Geometry check sheet. Reference: drawing and pictorial views, mm from the part's lowest x, y, z. A direction names the side the tool comes from. Coordinates: 2 decimals unless noted, no trailing zeros. Loops run counter-clockwise (first coordinate to the right, second up) from the corner with the lowest first, then second, coordinate; pieces in that order, holes last. Notation, with made-up numbers: (12.25, 54) - (60.25, 54) arc R22 cw to (60.25, 71) - close; hole circle Ø2 at (-23.5, 66.25). An arc over 180 degrees is marked (long way). One line per item, written item: value.
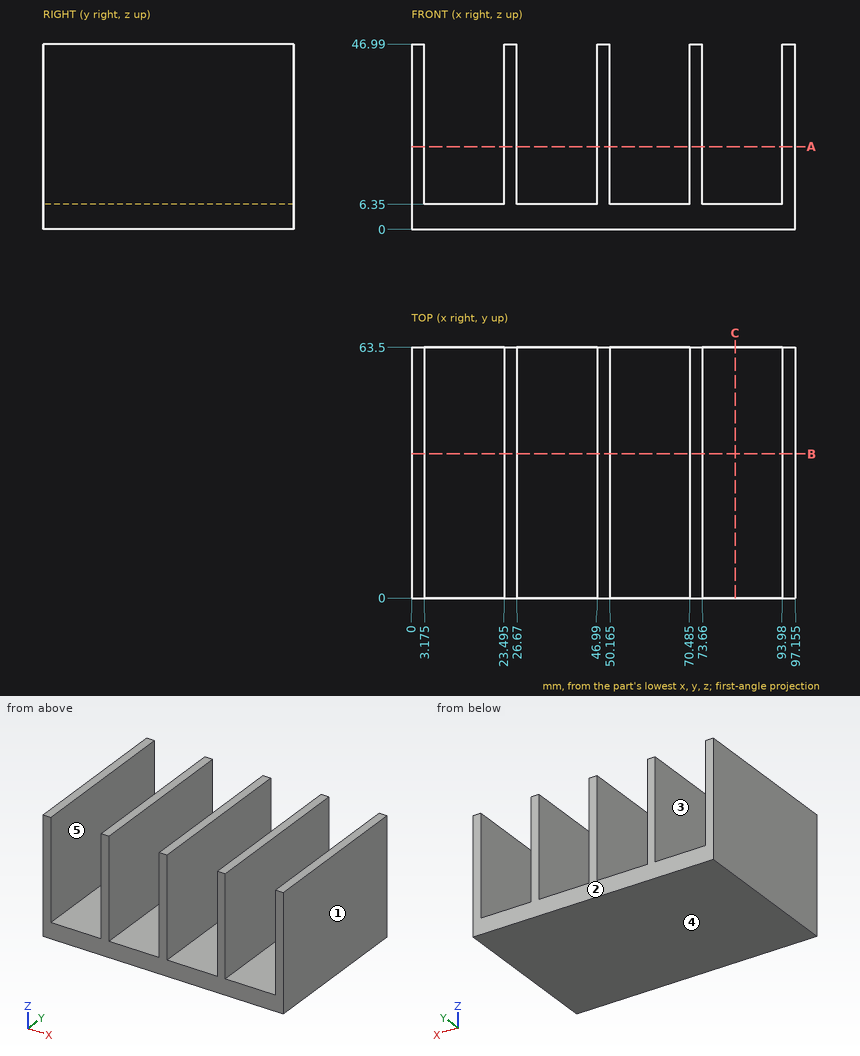
(1) Go/stop test with a flat-tipped pin: pin 1 Ø5 at (x, y) = (14.5, 28) entering from +Z. Record where the tip stops, or that it passes through.
Reply:
pin 1: z = 6.35
(2) Access from +Z, -Z, +X, -X, +Y, -Y to the whole of each face (thin tool, end or side, straight path). Record for the marked faces 4 and 5.
Reply:
face 4: -Z, +X, -X, +Y, -Y
face 5: +Z, +Y, -Y
(3) Material ranges on probe 1 along X at (y, z) = (31.5, 33) (3 decimals); probe 2 along Z at (x, y) = (42.5, 20.5), recorded low to high. Write a range as from..to.
Reply:
probe 1: 0..3.175, 23.495..26.67, 46.99..50.165, 70.485..73.66, 93.98..97.155
probe 2: 0..6.35
(4) Cross-section at B-B on y = 36.5. Record the cut outline in (x, z) (3 decimals), and give its area (3 significant figures).
Reply:
outline: (0, 0) - (97.155, 0) - (97.155, 46.99) - (93.98, 46.99) - (93.98, 6.35) - (73.66, 6.35) - (73.66, 46.99) - (70.485, 46.99) - (70.485, 6.35) - (50.165, 6.35) - (50.165, 46.99) - (46.99, 46.99) - (46.99, 6.35) - (26.67, 6.35) - (26.67, 46.99) - (23.495, 46.99) - (23.495, 6.35) - (3.175, 6.35) - (3.175, 46.99) - (0, 46.99) - close
area: 1,260 mm2
(5) Release check for a two-part mould opening along X. For the marked faces 1, 2 and 3 record: pulls with the +X half, pulls with the -X half, needs draft (parallel to the pull), parting line crosses it, or undercut.
Reply:
face 1: pulls with the +X half
face 2: needs draft
face 3: undercut
(6) Cross-section at A-A on z = 21. Record the cut outline in (x, y) (3 decimals), and give its area (3 significant figures).
Reply:
outline: (0, 0) - (3.175, 0) - (3.175, 63.5) - (0, 63.5) - close; (23.495, 0) - (26.67, 0) - (26.67, 63.5) - (23.495, 63.5) - close; (46.99, 0) - (50.165, 0) - (50.165, 63.5) - (46.99, 63.5) - close; (70.485, 0) - (73.66, 0) - (73.66, 63.5) - (70.485, 63.5) - close; (93.98, 0) - (97.155, 0) - (97.155, 63.5) - (93.98, 63.5) - close
area: 1,010 mm2
(7) Cross-section at C-C on x = 82. Record the cut outline in (y, z), and give its area (3 significant figures).
Reply:
outline: (0, 0) - (63.5, 0) - (63.5, 6.35) - (0, 6.35) - close
area: 403 mm2
